```python
from build123d import *

# Parameters (mm, degrees)
F0_W           = 50
F0_H           = 40
F1_DEPTH       = 20
F3_D           = 8.8
F3_CBORE_D     = 14.25
F3_CBORE_DEPTH = 8
F4_SIZE        = 0.5


with BuildPart() as f1:
    # F0 (on Top) → F1 (new body)
    with BuildSketch(Plane.XY):
        Rectangle(F0_W, F0_H)
    extrude(amount=F1_DEPTH)

    # F3 (through all)
    with Locations(Plane.XY.offset(20)):
        with Locations((0, 0)):
            CounterBoreHole(F3_D / 2, F3_CBORE_D / 2, F3_CBORE_DEPTH)

    # F4
    f4_edges = [f1.edges().sort_by_distance(p)[0] for p in [
        (25, 0, 20),
        (0, -20, 20),
        (0, 20, 20),
        (-25, 0, 20),
        (-7.125, 0, 20),
        (-25, 20, 10),
        (-25, -20, 10),
        (-25, 0, 0),
        (25, 20, 10),
        (0, 20, 0),
        (25, -20, 10),
        (0, -20, 0),
        (25, 0, 0),
    ]]
    chamfer(f4_edges, length=F4_SIZE)


solid = f1.part
```
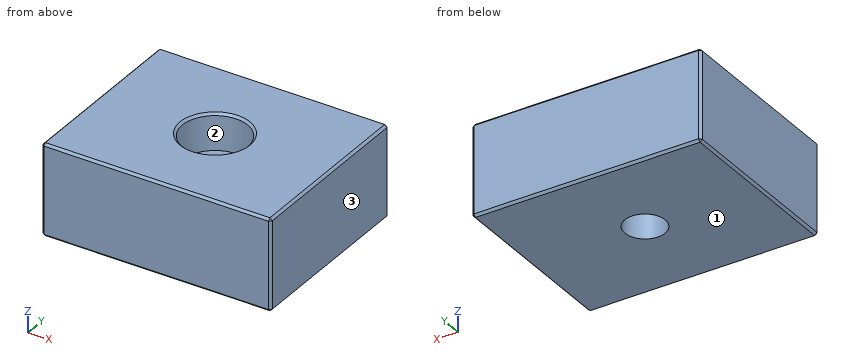
Model file for the job. Use its own axes, mm. Face numbers are marked on the shaded views. Coordinates: 2 decimals unless noted, no trailing zeros. Write each loop counter-clockwise with the first axis right and the second up, starting at its lowest first coordinate (ties: lowest second). Pieces come first, ordered by that corner, then holes. Notation, with made-up numbers: (61.25, 72.5) - (113.25, 72.5) arc R20 cw to (113.25, 81.5) - close; hole circle Ø1 at (59, -22.5). An arc over 180 degrees is marked (long way). One line per question, with ' | ' between items. Start each with the question number.
Q1. Cut at A-A, the plane y = 0. List the corners of the cut face in (x, z) (3 decimals).
Q2. Cut at B-B, the plane x = 0. List the corners of the cut face in (y, z) (3 decimals).
Q3. Pull direction X, two halves, no side cores. Call the marked faces 1, 2 and 3: pulls with the +X half, pulls with the -X half, needs draft (parallel to the pull), parting line crosses it, or undercut.
Q4. Drill centre lines: line 1 (Y direction, x = 0, z = 16.25) (3 decimals); line 2 (Y direction, x = 0, z = 2.75); line 3 (Z direction, x = -3.5, y = -5). Where is each one in solid material? Low to high. Write a range as [from, to].
Q5. Cut at C-C, the plane z = 7.5. List the corners of the cut face in (x, y).
Answer below:
1) outline: (-25, 0.5) - (-24.5, 0) - (-4.4, 0) - (-4.4, 12) - (-7.125, 12) - (-7.125, 19.5) - (-7.625, 20) - (-24.5, 20) - (-25, 19.5) - close; (4.4, 0) - (24.5, 0) - (25, 0.5) - (25, 19.5) - (24.5, 20) - (7.625, 20) - (7.125, 19.5) - (7.125, 12) - (4.4, 12) - close
2) outline: (-20, 0.5) - (-19.5, 0) - (-4.4, 0) - (-4.4, 12) - (-7.125, 12) - (-7.125, 19.5) - (-7.625, 20) - (-19.5, 20) - (-20, 19.5) - close; (4.4, 0) - (19.5, 0) - (20, 0.5) - (20, 19.5) - (19.5, 20) - (7.625, 20) - (7.125, 19.5) - (7.125, 12) - (4.4, 12) - close
3) face 1: needs draft | face 2: undercut | face 3: pulls with the +X half
4) line 1: [-20, -7.125], [7.125, 20] | line 2: [-20, -4.4], [4.4, 20] | line 3: [0, 12]
5) outline: (-25, -19.5) - (-24.5, -20) - (24.5, -20) - (25, -19.5) - (25, 19.5) - (24.5, 20) - (-24.5, 20) - (-25, 19.5) - close; hole circle Ø8.8 at (0, 0)
